from build123d import *

# Parameters (mm, degrees)
SKETCH_1_W                         = 192.5
SKETCH_1_H                         = 32
EXTRUDE_286_DEPTH                  = 34.5
SKETCH_4_W                         = 192.5
SKETCH_4_H                         = 13
EXTRUDE_1152_DEPTH                 = 1.5
CUT_EXTRUDE_1403_DEPTH             = 104.490639673
SKETCH_5_W                         = 192.5
SKETCH_5_H                         = 32
EXTRUDE_1554_DEPTH                 = 4
CUT_EXTRUDE_1876_DEPTH             = 198.261881771
CUT_EXTRUDE_2071_REACH             = 107.452
CUT_EXTRUDE_2071_DIRECTION_2_DEPTH = 106.451706956
FILLET_1_R                         = 2
PATTERN_LINEAR_1_COUNT             = 9
PATTERN_LINEAR_1_PITCH             = 17.5
FILLET_1_OF_PATTERN_LINEAR_1_R     = 2
HOLE_WIZARD_M5_D                   = 5.5
HOLE_WIZARD_M5_CSINK_D             = 10.4
HOLE_WIZARD_M5_CSINK_ANGLE         = 90
CHAMFER_1_SIZE                     = 2


with BuildPart() as part:
    # Эскиз1 → Extrude 286 (new body)
    with BuildSketch(Plane(origin=(0, 0, 0), x_dir=(1, 0, 0), z_dir=(0, 1, 0))):
        Rectangle(SKETCH_1_W, SKETCH_1_H)
    extrude(amount=EXTRUDE_286_DEPTH)

    # Эскиз4 → Extrude 1152 (add)
    with BuildSketch(Plane(origin=(0, 34.5, 0), x_dir=(1, 0, 0), z_dir=(0, 1, 0))):
        with Locations((0, 9.5)):
            Rectangle(SKETCH_4_W, SKETCH_4_H)
    extrude(amount=EXTRUDE_1152_DEPTH)

    # Эскиз2 → Cut-Extrude 1403 (cut, through all)
    with BuildSketch(Plane(origin=(0, 34.5, 0), x_dir=(1, 0, 0), z_dir=(0, 1, 0))):
        with BuildLine():
            Line((-84.75, -16), (-84.75, -6))
            ThreePointArc((-84.75, -6), (-78.75, 0), (-72.75, -6))
            Line((-72.75, -6), (-72.75, -16))
            Line((-72.75, -16), (-84.75, -16))
        make_face()
    cut_extrude_1403 = extrude(amount=-CUT_EXTRUDE_1403_DEPTH, mode=Mode.SUBTRACT)

    # Эскиз5 → Extrude 1554 (add)
    with BuildSketch(Plane(origin=(0, 36, 0), x_dir=(1, 0, 0), z_dir=(0, 1, 0))):
        Rectangle(SKETCH_5_W, SKETCH_5_H)
    extrude(amount=EXTRUDE_1554_DEPTH)

    # Эскиз3 → Cut-Extrude 1876 (cut, through all)
    with BuildSketch(Plane.ZY.offset(96.25)):
        Polygon((16, 33.25), (11, 34.5), (11, 36), (16, 37.25), align=None)
    extrude(amount=-CUT_EXTRUDE_1876_DEPTH, mode=Mode.SUBTRACT)

    # Эскиз7 → Cut-Extrude 2071 (cut, up to next)
    with BuildSketch(Plane(origin=(0, 40, 0), x_dir=(1, 0, 0), z_dir=(0, 1, 0)), mode=Mode.PRIVATE) as cut_extrude_2071_sk1:
        with BuildLine():
            Line((-83.75, -6), (-83.75, -16))
            Line((-83.75, -16), (-73.75, -16))
            Line((-73.75, -16), (-73.75, -6))
            ThreePointArc((-73.75, -6), (-78.75, -1), (-83.75, -6))
        make_face()
    cut_extrude_2071_tool1 = extrude(cut_extrude_2071_sk1.sketch, amount=-CUT_EXTRUDE_2071_REACH, mode=Mode.PRIVATE) & part.part
    cut_extrude_2071 = cut_extrude_2071_tool1.solids().sort_by_distance((-78.75, 40, 8.991792))[0]
    add(cut_extrude_2071, mode=Mode.SUBTRACT)

    # Эскиз7 → Cut-Extrude 2071 direction 2 (cut)
    with BuildSketch(Plane(origin=(0, 40, 0), x_dir=(1, 0, 0), z_dir=(0, 1, 0))):
        with BuildLine():
            Line((-83.75, -6), (-83.75, -16))
            Line((-83.75, -16), (-73.75, -16))
            Line((-73.75, -16), (-73.75, -6))
            ThreePointArc((-73.75, -6), (-78.75, -1), (-83.75, -6))
        make_face()
    cut_extrude_2071_direction_2 = extrude(amount=CUT_EXTRUDE_2071_DIRECTION_2_DEPTH, mode=Mode.SUBTRACT)

    # Скругление1
    fillet_1_edges = [part.edges().sort_by_distance(p)[0] for p in [
        (-72.75, 16.625, 16),
        (-84.75, 16.625, 16),
        (-83.75, 38.625, 16),
        (-73.75, 38.625, 16),
    ]]
    fillet(fillet_1_edges, radius=FILLET_1_R)

    # Линейный массив1: Cut-Extrude 1403, Cut-Extrude 2071, Cut-Extrude 2071 direction 2 ×9
    with Locations(*[(i * PATTERN_LINEAR_1_PITCH, 0, 0) for i in range(1, PATTERN_LINEAR_1_COUNT)]):
        add(cut_extrude_1403, mode=Mode.SUBTRACT)
        add(cut_extrude_2071, mode=Mode.SUBTRACT)
        add(cut_extrude_2071_direction_2, mode=Mode.SUBTRACT)

    # Скругление1 of Линейный массив1
    fillet_1_of_pattern_linear_1_edges = [part.edges().sort_by_distance(p)[0] for p in [
        (-55.25, 16.625, 16),
        (-67.25, 16.625, 16),
        (-66.25, 38.625, 16),
        (-56.25, 38.625, 16),
        (-37.75, 16.625, 16),
        (-49.75, 16.625, 16),
        (-48.75, 38.625, 16),
        (-38.75, 38.625, 16),
        (-20.25, 16.625, 16),
        (-32.25, 16.625, 16),
        (-31.25, 38.625, 16),
        (-21.25, 38.625, 16),
        (-2.75, 16.625, 16),
        (-14.75, 16.625, 16),
        (-13.75, 38.625, 16),
        (-3.75, 38.625, 16),
        (14.75, 16.625, 16),
        (2.75, 16.625, 16),
        (3.75, 38.625, 16),
        (13.75, 38.625, 16),
        (32.25, 16.625, 16),
        (20.25, 16.625, 16),
        (21.25, 38.625, 16),
        (31.25, 38.625, 16),
        (49.75, 16.625, 16),
        (37.75, 16.625, 16),
        (38.75, 38.625, 16),
        (48.75, 38.625, 16),
        (67.25, 16.625, 16),
        (55.25, 16.625, 16),
        (56.25, 38.625, 16),
        (66.25, 38.625, 16),
    ]]
    fillet(fillet_1_of_pattern_linear_1_edges, radius=FILLET_1_OF_PATTERN_LINEAR_1_R)

    # Крепление - M5 (through all)
    with Locations(Plane(origin=(0, 40, 0), x_dir=(1, 0, 0), z_dir=(0, 1, 0))):
        with Locations((-85, 8), (0, 8), (85, 8), (42.5, 8), (-42.5, 8)):
            CounterSinkHole(HOLE_WIZARD_M5_D / 2, HOLE_WIZARD_M5_CSINK_D / 2, counter_sink_angle=HOLE_WIZARD_M5_CSINK_ANGLE)

    # Фаска1
    chamfer_1_edges = [part.edges().sort_by_distance(p)[0] for p in [
        (0, 40, -16),
    ]]
    chamfer(chamfer_1_edges, length=CHAMFER_1_SIZE)


solid = part.part
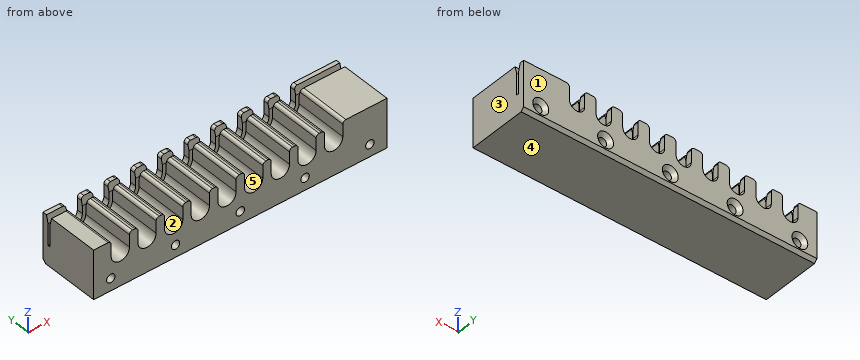
For this review, take the finished solid that the model builds, in its own axes (mm). Face numbers are marked on the shaded views. A direction names the side the tool comes from. Coordinates: 2 decimals unless noted, no trailing zeros. Order: outer loops, then holes, each group sorted by start corner. A loop starts at its lowest first (then second) coordinate and runs counter-clockwise, first axis right, second up. Notation, with made-up numbers: (31.5, 67) - (51.5, 67) arc R28 ccw to (51.5, 99) - close; hole circle Ø11 at (77, 65.5). An arc over 180 degrees is marked (long way). Answer as CSV lines item,"result". Start each with the question number.
1) Add section B-B (x = 42.5). State the section outline as (y, z) points.
2) Draft analysis for pull direction X (two halves, no side actions). For the marked faces 1, 2 and 3, state which applies: +X half, -X half, draft (parallel to the pull), parting line (faces both ways), or undercut.
3) Insertion check: P1, Ø2, axis at x = -41.5, y = 17, coming from the +Z side; P2, Ø3.5, axis at x = 85, z = -8, coming from the +Y side. Each pin has a flat end and moves straight along its axis. Give the tip position at first contact, or say it passes through.
4) To check wall thickness, follow line 1 along Z through (x, y) = (0, 23); line 2 along Y through (x, z) = (48.5, -2.5); line 3 along X through (y, z) = (11, -6). State the ranges of each line that lie inside material, in increasing order. Write a range as [from, to].
5) Add section D-D (x = 78). State the section outline as (y, z) points.
6) Add section A-A (x = -26.25). State the section outline as (y, z) points, then the cut area to 4 significant figures.
7) Add section C-C (y = 28.5). Count the separate pieces of the cut face and the enclosed holes in it, then the cut area to 3 significant figures.
8) Machinability: for the marked faces 4 and 5, which of the approach directions +Z, -Z, +X, -X, +Y, -Y give a long, thin tool a straight path to every point of the face, cutting with its end or side? Answer none if there is none.
Result:
1,outline,"(0, -16) - (38, -16) - (40, -14) - (40, -13.2) - (37.55, -10.75) - (0, -10.75) - close; (0, -5.25) - (37.55, -5.25) - (40, -2.8) - (40, 1.16) - (36, 1.16) - (36, -3) - (34.5, -3) - (34.5, 0.13) - (0, 0.13) - close"
2,face 1,"draft"
2,face 2,"undercut"
2,face 3,"+X half"
3,P1,"z = 0.96"
3,P2,"through"
4,line 1,"[-16, -10.75], [-5.25, 16]"
4,line 2,"[0, 34.5], [36, 40]"
4,line 3,"[-96.25, -86.89], [-83.11, -44.39], [-40.61, -1.89], [1.89, 40.61], [44.39, 83.11], [86.89, 96.25]"
5,outline,"(0, -16) - (38, -16) - (40, -14) - (40, 16) - (37.25, 16) - (36, 11) - (36, -3) - (34.5, -3) - (34.5, 11) - (33.25, 16) - (0, 16) - close"
6,outline,"(0, -16) - (38, -16) - (40, -14) - (40, 1) - (36, 1) - (36, -3) - (34.5, -3) - (34.5, 0) - (0, 0) - close"
6,area,"637.5 mm^2"
7,separate pieces,"1"
7,enclosed holes,"5"
7,area,"4,440 mm^2"
8,face 4,"-Z, +X, -X, +Y, -Y"
8,face 5,"+Z, -Y"
